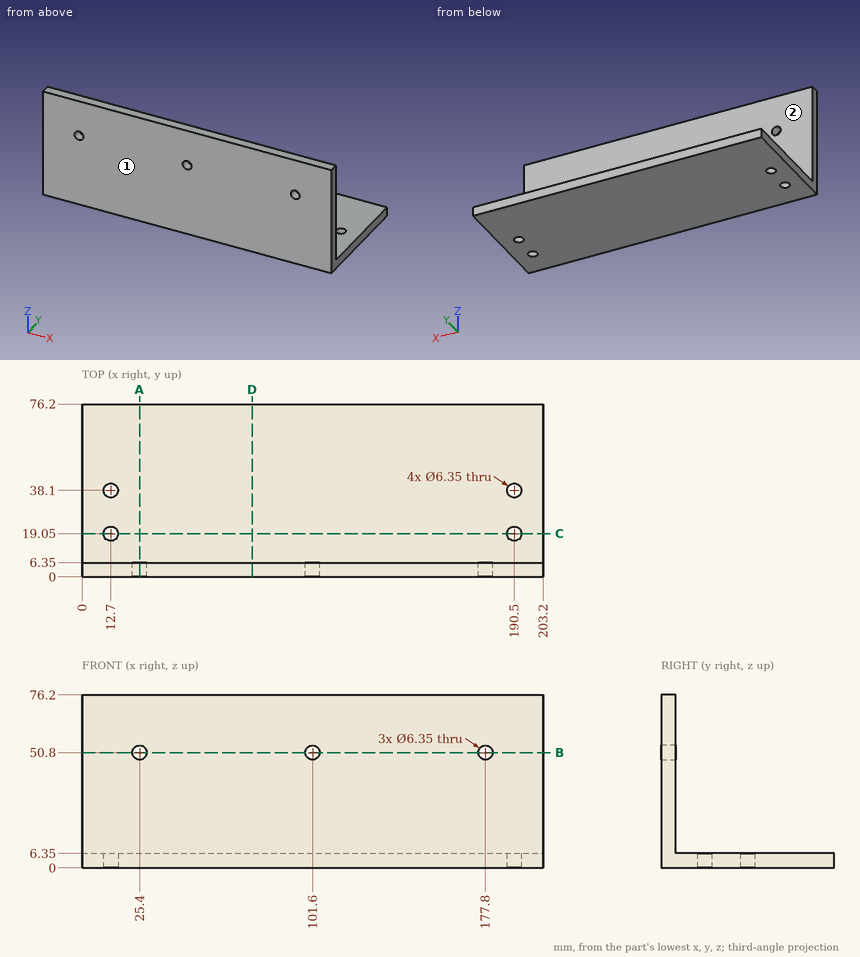
Part print with two shaded views. Sizes in mm from the minimum x, y, z corner. A direction names the side the tool comes from. Coordinates: 2 decimals unless noted, no trailing zeros. Write each loop counter-clockwise with the first axis right and the second up, starting at its lowest first coordinate (ties: lowest second). Pieces come first, ordered by that corner, then holes.
1. 3-axis set-ups, long thin cutter, end or side, ignore diameter. For the marked faces 1 and 2: which of +Z, -Z, +X, -X, +Y, -Y reach the whole face in a straight line?
Answer block:
face 1: +Z, -Z, +X, -X, -Y
face 2: +Z, +X, -X, +Y
2. Band-saw the part on D-D, the plane x = 75. Give the cut face in (y, z).
Answer block:
outline: (0, 0) - (76.2, 0) - (76.2, 6.35) - (6.35, 6.35) - (6.35, 76.2) - (0, 76.2) - close
3. Drill centre lines: probe 1 along X at (y, z) = (38, 3); probe 2 along X at (y, z) = (4.25, 50.8) (3 decimals); probe 3 along Y at (x, z) = (190, 2). Where is each one in solid material? Low to high.
Answer block:
probe 1: x = 0 to 9.53, 15.87 to 187.33, 193.67 to 203.2
probe 2: x = 0 to 22.225, 28.575 to 98.425, 104.775 to 174.625, 180.975 to 203.2
probe 3: y = 0 to 15.91, 22.19 to 34.96, 41.24 to 76.2
4. Drop flat-ended pins along their axis: pin 1 (21 mm diameter, centred on x = 53.5, y = 41.5, fed in from +Z); pin 2 (21 mm diameter, centred on x = 78.5, z = 49.5, fed in from +Y). Give the stop position or say it passes through.
Answer block:
pin 1: stops at z = 6.35
pin 2: stops at y = 6.35
5. Band-saw the part on A-A, the plane x = 25.4. Give the cut face in (y, z) (3 decimals), and give its area (3 significant figures).
Answer block:
outline: (0, 0) - (76.2, 0) - (76.2, 6.35) - (6.35, 6.35) - (6.35, 47.625) - (0, 47.625) - close; (0, 53.975) - (6.35, 53.975) - (6.35, 76.2) - (0, 76.2) - close
area: 887 mm2
6. Band-saw the part on C-C, the plane y = 19.05. Give the cut face in (x, z) (3 decimals).
Answer block:
outline: (0, 0) - (9.525, 0) - (9.525, 6.35) - (0, 6.35) - close; (15.875, 0) - (187.325, 0) - (187.325, 6.35) - (15.875, 6.35) - close; (193.675, 0) - (203.2, 0) - (203.2, 6.35) - (193.675, 6.35) - close
7. Band-saw the part on B-B, the plane z = 50.8. Give the cut face in (x, y) (3 decimals), and give its area (3 significant figures).
Answer block:
outline: (0, 0) - (22.225, 0) - (22.225, 6.35) - (0, 6.35) - close; (28.575, 0) - (98.425, 0) - (98.425, 6.35) - (28.575, 6.35) - close; (104.775, 0) - (174.625, 0) - (174.625, 6.35) - (104.775, 6.35) - close; (180.975, 0) - (203.2, 0) - (203.2, 6.35) - (180.975, 6.35) - close
area: 1,170 mm2
